Autodesk Inventor part; units mm, degrees
ref_plane "YZ Plane" through (0, 0, 0) normal (1, 0, 0) x (0, 1, 0)
ref_plane "XZ Plane" through (0, 0, 0) normal (0, 1, 0) x (-1, 0, 0)
ref_plane "XY Plane" through (0, 0, 0) normal (0, 0, 1) x (1, 0, 0)
sketch "Sketch1" plane through (0, 0, 0) normal (0, 0, 1) x (1, 0, 0)
  line L0 (-5.591, -7.5) -> (-5.591, 7.5)
  line L1 (-5.591, 7.5) -> (5.591, 7.5)
  line L2 (5.591, 7.5) -> (5.591, -7.5)
  line L3 (5.591, -7.5) -> (-5.591, -7.5)
  line L4 (-5.591, -7.5) -> (5.591, 7.5) construction
  line L5 (-5.591, 7.5) -> (5.591, -7.5) construction
  point P0 (0, 0)
  dimension "d0" = 15
  dimension "d1" = 11.182
extrude "Extrusion1" add sketch "Sketch1" along normal blind 133
sketch "Sketch2" plane through (0, 0, 133) normal (0, 0, 1) x (1, 0, 0)
  line L0 (-5.591, 7.5) -> (-5.591, -7.5)
  line L1 (-5.591, 0) -> (-5.591, -5)
  line L2 (-5.591, -5) -> (1.909, -5)
  line L3 (1.909, -5) -> (1.909, 5)
  line L4 (5.591, 7.5) -> (-5.591, 7.5)
  line L5 (1.909, 5) -> (-5.591, 5)
  line L6 (-5.591, 5) -> (-5.591, 0)
  point P0 (0, 0)
  dimension "d4" = 5
  dimension "d5" = 7.5
  dimension "d6" = 10
  dimension "d7" = 7.5
extrude "Extrusion2" add sketch "Sketch2" along normal blind 6.5
ref_plane "Work Plane1" through (0, 0, 66.5) normal (0, 0, 1) x (1, 0, 0)
mirror "Mirror1" about plane through (0, 0, 66.5) normal (0, 0, 1) of "Extrusion2"
sketch "Sketch3" plane through (-5.591, -7.5, 0) normal (0, -1, 0) x (1, 0, 0)
  line L0 (0, 133) -> (11.182, 133)
  line L1 (11.182, 133) -> (6.182, 133)
  line L2 (6.182, 133) -> (5.591, 0)
  line L3 (11.182, 0) -> (0, 0)
  line L4 (5.591, 0) -> (11.182, 0)
  line L5 (11.182, 0) -> (11.182, 133)
  line L6 (11.182, 0) -> (11.182, 133)
  line L7 (0, 0) -> (0, 133)
  dimension "d10" = 5
extrude "Extrusion3" add sketch "Sketch3" along normal blind 5 contours L0 L5 L3 L2
sketch "Sketch4" plane through (0, 0, 139.5) normal (0, 0, 1) x (1, 0, 0)
  line L0 (-5.591, 5) -> (-5.591, -5)
  line L1 (-5.591, -5) -> (1.909, -5)
  line L2 (1.909, -5) -> (1.909, 5)
  line L3 (1.909, 5) -> (-5.591, 5)
  line L4 (-5.191, -4.6) -> (-5.191, 4.6)
  line L5 (-5.191, 4.6) -> (1.509, 4.6)
  line L6 (1.509, 4.6) -> (1.509, -4.6)
  line L7 (1.509, -4.6) -> (-5.191, -4.6)
  point P0 (0, 0)
  dimension "d13" = 0.4
extrude "Extrusion4" cut sketch "Sketch4" against normal up to surface (6.5 mm away)
mirror "Mirror2" about plane through (0, 0, 66.5) normal (0, 0, 1) of "Extrusion4"
ref_plane "Work Plane2" through (0, 0, 66.5) normal (0, 0, 1) x (1, 0, 0)
properties part number "Lower Beam Support"
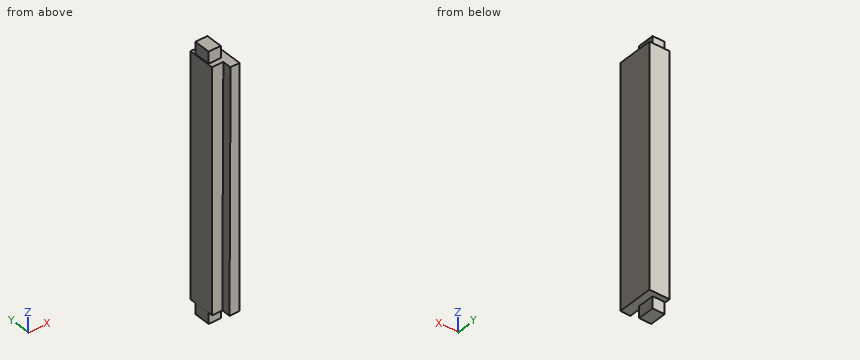
For this review, take the finished solid that the model builds, in its own axes (mm). Coordinates: 2 decimals unless noted, no trailing zeros. Loops run counter-clockwise (first coordinate to the right, second up) from the corner with the lowest first, then second, coordinate; pieces in that order, holes last. Notation, with made-up numbers: (60, 40.25) - (88, 40.25) arc R32 ccw to (88, 66.25) - close; hole circle Ø10 at (-33.5, 88). An arc over 180 degrees is marked (long way). Use one line per item in the form item = value. Start each with the question number.
1) Take a section at D-D (y = -10). State the section outline as (x, z) points.
2) Take a section at A-A (y = -2.75). State the section outline as (x, z) points.
3) Take a section at B-B (z = 127). State the section outline as (x, y) points, plus the area to 3 significant figures.
4) To check wall thickness, follow probe 1 along Y at (x, z) = (-1.25, 95); probe 2 along Z at (x, y) = (-4.5, -5.75); probe 3 along X at (y, z) = (-9.5, 101). State the ranges of each line that lie inside material, in increasing order. Write a range as from..to.
5) For pin 1 (3 mm diameter, centred on x = -3, z = -2.5, fed in from -Y); pin 2 (7 mm diameter, centred on y = 0, z = 137, fed in from -X); pin 3 (3 mm diameter, centred on x = -1.5, z = -3.5, fed in from +Y); pin 4 (5 mm diameter, centred on x = -0.5, y = -5.5, fed in from -Z), all flat-tipped, find the tip position at first contact; note any pin that passes through.
6) Take a section at C-C (x = 2.75). State the section outline as (y, z) points.
From the geometry:
q1.outline = (0, 0) - (5.59, 0) - (5.59, 133) - (0.59, 133) - close
q2.outline = (-5.59, 0) - (-5.19, 0) - (-5.19, -6.5) - (1.51, -6.5) - (1.51, 0) - (5.59, 0) - (5.59, 133) - (1.51, 133) - (1.51, 139.5) - (-5.19, 139.5) - (-5.19, 133) - (-5.59, 133) - close
q3.outline = (-5.59, -7.5) - (0.56, -7.5) - (0.56, -12.5) - (5.59, -12.5) - (5.59, 7.5) - (-5.59, 7.5) - close
q3.area = 193 mm2
q4.probe_1 = -7.5..7.5
q4.probe_2 = 0..133
q4.probe_3 = 0.45..5.59
q5.pin_1 = -4.6
q5.pin_2 = -5.19
q5.pin_3 = 4.6
q5.pin_4 = -6.5
q6.outline = (-12.5, 0) - (7.5, 0) - (7.5, 133) - (-12.5, 133) - close
